Part model, mm, in its own coordinate system. A direction names the side the tool comes from. Round coordinates to 2 decimals unless told otherwise and drop trailing zeros. Write each loop counter-clockwise with the first axis right and the second up, starting at its lowest first coordinate (ties: lowest second). Pieces come first, ordered by that corner, then holes. Notation, with made-up numbers: (-6, 15) -> (29, 15) arc R17 ccw to (29, 21) -> close; hole circle Ø5 at (-28.75, 24). An arc over 180 degrees is marked (long way). Return JSON: item names as keys, results as strings. Group by question number.
```python
from build123d import *

# Parameters (mm, degrees)
SKETCH_1_R          = 8
SKETCH_1_R_2        = 2.6
EXTRUDE_1_DEPTH     = 18
SKETCH_2_R          = 25
SKETCH_2_R_2        = 1.6
EXTRUDE_2_DEPTH     = 4
SKETCH_4_R          = 2.4
CUT_EXTRUDE_1_DEPTH = 10
SKETCH_5_R          = 2.6
CUT_EXTRUDE_2_DEPTH = 10


with BuildPart() as part:
    # 草图1 → 凸台-拉伸1 (new body)
    with BuildSketch(Plane(origin=(0, 0, 0), x_dir=(1, 0, 0), z_dir=(0, 1, 0))):
        with Locations(Location((0, 0, 0), (0, 0, 270))):
            Circle(SKETCH_1_R)
        with Locations(Location((0, 0, 0), (0, 0, 270))):
            Circle(SKETCH_1_R_2, mode=Mode.SUBTRACT)
    extrude(amount=EXTRUDE_1_DEPTH)

    # 草图2 → 凸台-拉伸2 (add)
    with BuildSketch(Plane(origin=(0, 18, 0), x_dir=(1, 0, 0), z_dir=(0, 1, 0))):
        with Locations(Location((0, 0, 0), (0, 0, 270))):
            Circle(SKETCH_2_R)
        with Locations(Location((16, 0, 0), (0, 0, 270))):
            Circle(SKETCH_2_R_2, mode=Mode.SUBTRACT)
        with Locations(Location((8, -13.856406461, 0), (0, 0, 270))):
            Circle(SKETCH_2_R_2, mode=Mode.SUBTRACT)
        with Locations(Location((-8, -13.856406461, 0), (0, 0, 270))):
            Circle(SKETCH_2_R_2, mode=Mode.SUBTRACT)
        with Locations(Location((-16, 0, 0), (0, 0, 270))):
            Circle(SKETCH_2_R_2, mode=Mode.SUBTRACT)
        with Locations(Location((-8, 13.856406461, 0), (0, 0, 270))):
            Circle(SKETCH_2_R_2, mode=Mode.SUBTRACT)
        with Locations(Location((8, 13.856406461, 0), (0, 0, 270))):
            Circle(SKETCH_2_R_2, mode=Mode.SUBTRACT)
    extrude(amount=EXTRUDE_2_DEPTH)

    # 草图4 → 切除-拉伸1 (cut)
    with BuildSketch(Plane.XY):
        with Locations(Location((0, 10, 0), (0, 0, 90))):
            Circle(SKETCH_4_R)
    extrude(amount=-CUT_EXTRUDE_1_DEPTH, mode=Mode.SUBTRACT)

    # 草图5 → 切除-拉伸2 (cut)
    with BuildSketch(Plane.XZ.offset(-18)):
        with Locations(Location((0, 0, 0), (0, 0, 90))):
            Circle(SKETCH_5_R)
    extrude(amount=-CUT_EXTRUDE_2_DEPTH, mode=Mode.SUBTRACT)


solid = part.part
```
Item 1: Two-plate mould, pull along X, no slides. Class faces 3 (the face through (6, 18, -6)), 4 (the face through (8.07, 19.972, -15.455)), 5 (the face through (-3.06, 8.87, 7.39)): released by +X, released by -X, zero draft, split by the parting line, or undercut.
Item 2: Cut at B-B (x = 16). Write the cut outline in (y, z).
Item 3: Cut at A-A (z = -13). Write the cut outline in (x, y), then the cut area to 3 significant figures.
Item 4: Cut at C-C (z = -6). Write the cut outline in (x, y).
Item 5: Flat gauge pins, fed straight in: P1, Ø1.9, axis at x = 16, z = 0, coming from the -Y side; P2, Ø12, axis at y = 17.5, z = 0.5, coming from the +X side; P3, Ø6, axis at x = 8, y = 8, coming from the +Z side (3 decimals); P4, Ø10, axis at x = 0, z = -19.5, coming from the -Y side. Where does each tip first touch, or does it go through?
Item 6: Cut at D-D (y = 15.5). Write the cut outline in (x, z).
Item 7: Which spindle directions (+Z, -Z, +X, -X, +Y, -Y) get a long thin tool onto all of the face, cutting with end or side? Do faces 1 (the face through (-1.62, 8.23, -5.23)), 2 (the face through (-14.414, 19.972, -0.208)). Say none if no direction does.
Item 8: Wall check: L1, parallel to X at y = 19.9, z = 0; L2, parallel to Y at x = -9, z = -2; L3, parallel to Z at x = 17, y = 19.75. Give the ranges that are in metal, low to high.
Checks:
{
 "1": {"face 3": "zero draft", "face 4": "undercut", "face 5": "split by the parting line"},
 "2": {"outline": "(18, -19.21) -> (22, -19.21) -> (22, -1.6) -> (18, -1.6) -> close; (18, 1.6) -> (22, 1.6) -> (22, 19.21) -> (18, 19.21) -> close"},
 "3": {"outline": "(-21.35, 18) -> (-9.35, 18) -> (-9.35, 22) -> (-21.35, 22) -> close; (-6.65, 18) -> (6.65, 18) -> (6.65, 22) -> (-6.65, 22) -> close; (9.35, 18) -> (21.35, 18) -> (21.35, 22) -> (9.35, 22) -> close", "area": "149 mm2"},
 "4": {"outline": "(-24.27, 18) -> (-5.29, 18) -> (-5.29, 0) -> (5.29, 0) -> (5.29, 18) -> (24.27, 18) -> (24.27, 22) -> (-24.27, 22) -> close; hole circle Ø4.8 at (0, 10)"},
 "5": {"P1": "passes through", "P2": "stops at x = 25", "P3": "stops at z = 6.245", "P4": "stops at y = 18"},
 "6": {"outline": "circle Ø16 at (0, 0); hole circle Ø5.2 at (0, 0)"},
 "7": {"face 1": "-Z", "face 2": "+Y, -Y"},
 "8": {"L1": "x = -25 to -17.6, -14.4 to -2.6, 2.6 to 14.4, 17.6 to 25", "L2": "y = 18 to 22", "L3": "z = -18.33 to -1.25, 1.25 to 18.33"}
}
